Geometry check sheet. Reference: the model listing, model coordinates, mm. Face numbers are marked on the shaded views. Give positions to 0.01 mm unless a question says otherwise; leave off trailing zeros. Order: outer loops, then holes, each group sorted by start corner. A loop starts at its lowest first (then second) coordinate and runs counter-clockwise, first axis right, second up. Notation, with made-up numbers: M -31.5,76.5 L 1.5,76.5 A29 ccw 1.5,103.5 Z; hole C 5.25,19.5 d5. An arc over 180 degrees is marked long. Answer as CSV lines item,"result". Start each with the question number.
Q1. Go/stop test with flat-tipped pins: pin 1 (3 mm diameter, centred on x = -5.5, y = -19, fed in from -Z); pin 2 (0.6 mm diameter, centred on y = -22.5, z = 3, fed in from -X); pin 3 (2 mm diameter, centred on y = -9.5, z = 1.5, fed in from -X); pin 4 (1.4 mm diameter, centred on y = 0.5, z = 3.5, fed in from +X). Record where each tip stops, or that it passes through.
Q2. Section check A-A, the plane x = 0. Record the boundary of the cut face in (y, z).
Q3. Thickness scan on line 1 (Z direction, x = -13, y = 18); line 2 (Y direction, x = 22, z = 2.55); line 3 (X direction, y = 10, z = 0.2). Record the ranges inside material, lowest first.
Q4. Mould release check, pull along X, two halves, no side actions. Record for the marked faces 1 and 2: +X half, -X half, draft (parallel to the pull), parting line (faces both ways), or undercut.
```python
from build123d import *

# Parameters (mm, degrees)
F0_R     = 27
F0_R_2   = 19.25
F1_DEPTH = 2.5
F2_W     = 5
F2_H     = 5
F3_DEPTH = 2
F4_R     = 0.75
F5_R     = 1.5


with BuildPart() as f1:
    # F0 (on Top) → F1 (new body)
    with BuildSketch(Plane.XY):
        Circle(F0_R)
        Circle(F0_R_2, mode=Mode.SUBTRACT)
    extrude(amount=F1_DEPTH)

    # F2 (on face) → F3 (join)
    with BuildSketch(Plane.XY.offset(2.5)):
        with Locations((23, 0)):
            Rectangle(F2_W, F2_H)
        Polygon((19.79899, 16.263456), (16.263456, 19.79899), (12.727922, 16.263456), (16.263456, 12.727922), align=None)
        with Locations((0, 23)):
            Rectangle(F2_W, F2_H)
        Polygon((-16.263456, 19.79899), (-19.79899, 16.263456), (-16.263456, 12.727922), (-12.727922, 16.263456), align=None)
        with Locations((-23, 0)):
            Rectangle(F2_W, F2_H)
        Polygon((-19.79899, -16.263456), (-16.263456, -19.79899), (-12.727922, -16.263456), (-16.263456, -12.727922), align=None)
        with Locations((0, -23)):
            Rectangle(F2_W, F2_H)
        Polygon((16.263456, -19.79899), (19.79899, -16.263456), (16.263456, -12.727922), (12.727922, -16.263456), align=None)
    extrude(amount=F3_DEPTH)

    # F4
    f4_edges = [f1.edges().sort_by_distance(p)[0] for p in [
        (-25.5, 0, 4.5),
        (-23, -2.5, 4.5),
        (-20.5, 0, 4.5),
        (-23, 2.5, 4.5),
        (-18.031223, 18.031223, 4.5),
        (-18.031223, 14.495689, 4.5),
        (-14.495689, 14.495689, 4.5),
        (-14.495689, 18.031223, 4.5),
        (0, 25.5, 4.5),
        (-2.5, 23, 4.5),
        (0, 20.5, 4.5),
        (2.5, 23, 4.5),
        (18.031223, 18.031223, 4.5),
        (14.495689, 18.031223, 4.5),
        (14.495689, 14.495689, 4.5),
        (18.031223, 14.495689, 4.5),
        (23, -2.5, 4.5),
        (25.5, 0, 4.5),
        (23, 2.5, 4.5),
        (20.5, 0, 4.5),
        (18.031223, -18.031223, 4.5),
        (18.031223, -14.495689, 4.5),
        (14.495689, -14.495689, 4.5),
        (14.495689, -18.031223, 4.5),
        (0, -25.5, 4.5),
        (2.5, -23, 4.5),
        (0, -20.5, 4.5),
        (-2.5, -23, 4.5),
        (-18.031223, -18.031223, 4.5),
        (-14.495689, -18.031223, 4.5),
        (-14.495689, -14.495689, 4.5),
        (-18.031223, -14.495689, 4.5),
    ]]
    fillet(f4_edges, radius=F4_R)

    # F5
    f5_edges = [f1.edges().sort_by_distance(p)[0] for p in [
        (-27, 0, 0),
    ]]
    fillet(f5_edges, radius=F5_R)


solid = f1.part
```
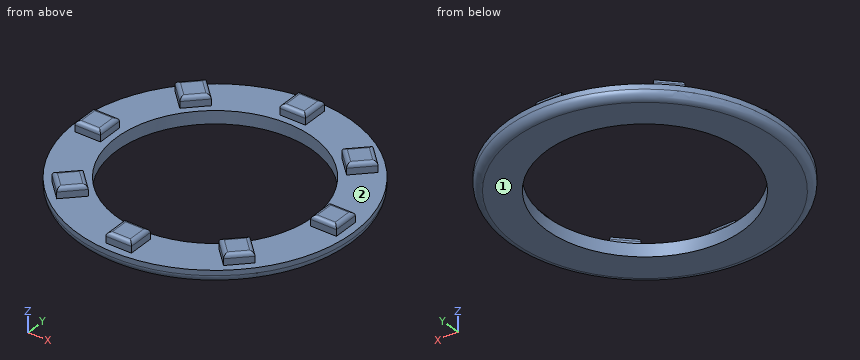
Answer block:
1,pin 1,"stops at z = 0"
1,pin 2,"stops at x = -2.5"
1,pin 3,"stops at x = -25.63"
1,pin 4,"stops at x = 25.5"
2,outline,"M -27,1.5 A1.5 ccw -25.5,0 L -19.25,0 L -19.25,2.5 L -20.5,2.5 L -20.5,3.75 A0.75 ccw -21.25,4.5 L -24.75,4.5 A0.75 ccw -25.5,3.75 L -25.5,2.5 L -27,2.5 Z; M 19.25,0 L 25.5,0 A1.5 ccw 27,1.5 L 27,2.5 L 25.5,2.5 L 25.5,3.75 A0.75 ccw 24.75,4.5 L 21.25,4.5 A0.75 ccw 20.5,3.75 L 20.5,2.5 L 19.25,2.5 Z"
3,line 1,"z = 0 to 2.5"
3,line 2,"y = -2.5 to 2.5"
3,line 3,"x = -24.27 to -16.45, 16.45 to 24.27"
4,face 1,"draft"
4,face 2,"undercut"
